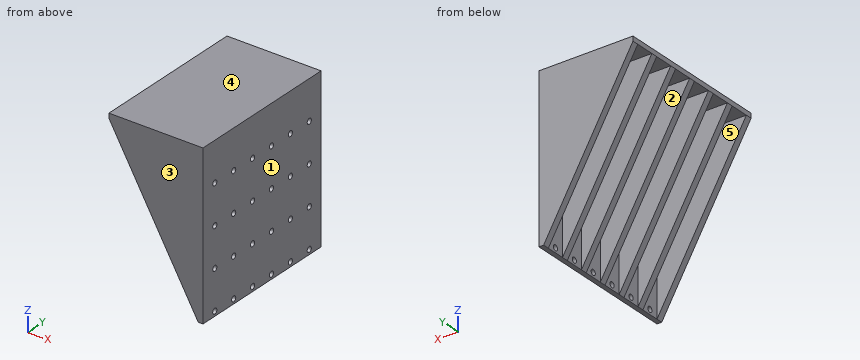
from build123d import *

# Parameters (mm, degrees)
BOSS_EXTRUDE1_DEPTH = 100
BOSS_EXTRUDE2_DEPTH = 4
LPATTERN1_COUNT     = 7
LPATTERN1_PITCH     = 16
SKETCH3_R           = 1.75
CUT_EXTRUDE1_DEPTH  = 10


with BuildPart() as part:
    # Sketch1 → Boss-Extrude1 (new body)
    with BuildSketch(Plane(origin=(0, 0, 0), x_dir=(1, 0, 0), z_dir=(0, 1, 0))):
        Polygon((0, 0), (-60, 0), (-60, 3), (-3, 3), (-3, 103), (0, 103), align=None)
    extrude(amount=BOSS_EXTRUDE1_DEPTH)

    # Sketch2 → Boss-Extrude2 (add)
    with BuildSketch(Plane(origin=(0, 100, 0), x_dir=(1, 0, 0), z_dir=(0, 1, 0))):
        Polygon((-60, 3), (-3, 103), (-3, 3), align=None)
    boss_extrude2 = extrude(amount=-BOSS_EXTRUDE2_DEPTH)

    # LPattern1: Boss-Extrude2 ×7
    with Locations(*[(0, -i * LPATTERN1_PITCH, 0) for i in range(1, LPATTERN1_COUNT)]):
        add(boss_extrude2)

    # Sketch3 → Cut-Extrude1 (cut)
    with BuildSketch(Plane(origin=(0, 0, 0), x_dir=(0, 0, -1), z_dir=(1, 0, 0))):
        with Locations((25, 10)):
            Circle(SKETCH3_R)
        with Locations((50, 10)):
            Circle(SKETCH3_R)
        with Locations((75, 10)):
            Circle(SKETCH3_R)
        with Locations((100, 10)):
            Circle(SKETCH3_R)
        with Locations((50, 26)):
            Circle(SKETCH3_R)
        with Locations((75, 26)):
            Circle(SKETCH3_R)
        with Locations((100, 26)):
            Circle(SKETCH3_R)
        with Locations((50, 42)):
            Circle(SKETCH3_R)
        with Locations((75, 42)):
            Circle(SKETCH3_R)
        with Locations((100, 42)):
            Circle(SKETCH3_R)
        with Locations((50, 58)):
            Circle(SKETCH3_R)
        with Locations((75, 58)):
            Circle(SKETCH3_R)
        with Locations((100, 58)):
            Circle(SKETCH3_R)
        with Locations((50, 74)):
            Circle(SKETCH3_R)
        with Locations((75, 74)):
            Circle(SKETCH3_R)
        with Locations((100, 74)):
            Circle(SKETCH3_R)
        with Locations((50, 90)):
            Circle(SKETCH3_R)
        with Locations((75, 90)):
            Circle(SKETCH3_R)
        with Locations((100, 90)):
            Circle(SKETCH3_R)
        with Locations((25, 26)):
            Circle(SKETCH3_R)
        with Locations((25, 42)):
            Circle(SKETCH3_R)
        with Locations((25, 58)):
            Circle(SKETCH3_R)
        with Locations((25, 74)):
            Circle(SKETCH3_R)
        with Locations((25, 90)):
            Circle(SKETCH3_R)
    extrude(amount=-CUT_EXTRUDE1_DEPTH, mode=Mode.SUBTRACT)


solid = part.part
Can you work these out from the model? Positions are in its coordinate system, mm. Face numbers are marked on the shaded views. A direction names the side the tool comes from. Coordinates: 2 decimals unless noted, no trailing zeros. Order: outer loops, then holes, each group sorted by start corner. A loop starts at its lowest first (then second) coordinate and runs counter-clockwise, first axis right, second up. Notation, with made-up numbers: (75.25, 34) - (121.25, 34) arc R14 cw to (121.25, 44) - close; hole circle Ø5 at (7, 63.5). An arc over 180 degrees is marked (long way). Answer as a JSON object with one key per item and string values. Group by question number.
Q1. Imagine slicing it at B-B (z = -69). Please give me the cut outline in (x, y).
Q2. Imagine slicing it at A-A (y = 42). Please give me the cut outline in (x, z), and give its area (3 significant figures).
Q3. I need wall thicknesses on line 1 (Z direction, x = -0.9, y = 90); line 2 (Z direction, x = -4.5, y = 94.5). Which ranges of each line are inside material? Lowest first, please. Write a range as from..to.
Q4. Imagine slicing it at C-C (z = -50). Give the number of separate pieces and of enclosed holes in the cut face, and give its area (3 significant figures).
Q5. Imagine slicing it at D-D (x = -45). Please give me the cut outline in (y, z).
Q6. Will these pins go through, and if not, where does the flat tip stop? P1, Ø5.5, axis at y = 74, z = -100, coming from the -X side; P2, Ø2, axis at y = 26, z = -75, coming from the -X side; P3, Ø8, axis at y = 78, z = -13, coming from the -X side; P4, Ø5, axis at x = -44, y = 50, coming from the -Z side.
Q7. We'd pull the mould along Y, two halves only. Please class the marked faces 3, 4 and 5: +Y half, -Y half, draft (parallel to the pull), parting line (faces both ways), or undercut.
Q8. On a 3-axis mill with a long thin cutter (end or side, diameter ignored), from which of +Z, -Z, +X, -X, +Y, -Y can I reach the whole of each face in a straight line? I mean the marked faces 1 and 2. Say none if no direction works.
Determined:
{
 "1": {"outline": "(-22.38, 0) - (0, 0) - (0, 100) - (-22.38, 100) - (-22.38, 96) - (-3, 96) - (-3, 84) - (-22.38, 84) - (-22.38, 80) - (-3, 80) - (-3, 68) - (-22.38, 68) - (-22.38, 64) - (-3, 64) - (-3, 52) - (-22.38, 52) - (-22.38, 48) - (-3, 48) - (-3, 36) - (-22.38, 36) - (-22.38, 32) - (-3, 32) - (-3, 20) - (-22.38, 20) - (-22.38, 16) - (-3, 16) - (-3, 4) - (-22.38, 4) - close"},
 "2": {"outline": "(-60, -3) - (-3, -3) - (-3, -23.25) - (0, -23.25) - (0, 0) - (-60, 0) - close; (-3, -103) - (0, -103) - (0, -101.75) - (-3, -101.75) - close; (-3, -98.25) - (0, -98.25) - (0, -76.75) - (-3, -76.75) - close; (-3, -73.25) - (0, -73.25) - (0, -51.75) - (-3, -51.75) - close; (-3, -48.25) - (0, -48.25) - (0, -26.75) - (-3, -26.75) - close", "area": "438 mm2"},
 "3": {"line 1": "z = -103..-101.75, -98.25..-76.75, -73.25..-51.75, -48.25..-26.75, -23.25..0", "line 2": "z = -3..0"},
 "4": {"separate pieces": "7", "enclosed holes": "0", "area": "1,080 mm2"},
 "5": {"outline": "(0, -29.32) - (4, -29.32) - (4, -3) - (16, -3) - (16, -29.32) - (20, -29.32) - (20, -3) - (32, -3) - (32, -29.32) - (36, -29.32) - (36, -3) - (48, -3) - (48, -29.32) - (52, -29.32) - (52, -3) - (64, -3) - (64, -29.32) - (68, -29.32) - (68, -3) - (80, -3) - (80, -29.32) - (84, -29.32) - (84, -3) - (96, -3) - (96, -29.32) - (100, -29.32) - (100, 0) - (0, 0) - close"},
 "6": {"P1": "stops at x = -3", "P2": "passes through", "P3": "stops at x = -56.27", "P4": "stops at z = -35.46"},
 "7": {"face 3": "-Y half", "face 4": "draft", "face 5": "undercut"},
 "8": {"face 1": "+Z, -Z, +X, +Y, -Y", "face 2": "-Z, -X"}
}
